Here's how the part is built. I have some questions about the finished solid (model axes, mm). A direction names the side the tool comes from. Coordinates: 2 decimals unless noted, no trailing zeros. Order: outer loops, then holes, each group sorted by start corner. A loop starts at its lowest first (then second) coordinate and runs counter-clockwise, first axis right, second up. Notation, with made-up numbers: (-26.75, 65.5) - (9.25, 65.5) arc R8 ccw to (9.25, 76.5) - close; hole circle Ø11 at (6, -33). An arc over 180 degrees is marked (long way). Answer as CSV lines item,"result". Start each with the question number.
Item 1: Imagine slicing it at D-D on x = -48. List the corners of the cut face in (y, z) for me.
Item 2: Imagine slicing it at C-C on z = -21. List the corners of the cut face in (x, y) for me (3 decimals), and give its area (3 significant figures).
Item 3: I need wall thicknesses on line 1 (X direction, y = -0.4, z = 0); line 2 (X direction, y = -0.65, z = -41); line 3 (Y direction, x = 40, z = -75.5). Which ranges of each line are inside material? Lowest first, please.
Item 4: On a 3-axis mill with a long thin cutter (end or side, diameter ignored), from which of +Z, -Z, +X, -X, +Y, -Y can I reach the whole of each face in a straight line? I mean faces 4 (the face through (83.647, -0.986, 7.831)), 5 (the face through (28.5, -1.49, -29.57)). Say none if no direction works.
Item 5: I'm going to push flat-ended pins straight in: pin 1 (0.8 mm diameter, centred on x = 22, z = -25, fed in from -Y) (3 decimals); pin 2 (12 mm diameter, centred on x = 11, z = -55.5, fed in from +Y); pin 3 (19 mm diameter, centred on x = -15.5, z = 22, fed in from -Y); pin 4 (0.5 mm diameter, centred on y = -1.5, z = 23, fed in from +X). Where does each tip first touch, or does it pass through?
Item 6: We'd pull the mould along Z, two halves only. Please class faces 1 (the face through (3.167, -0.986, -89.444)), 2 (the face through (7.509, -0.493, 23.846)), 3 (the face through (-28.57, -1.49, -29.5)): pulls with the +Z half, pulls with the -Z half, needs draft (parallel to the pull), parting line crosses it, or undercut.
Item 7: Imagine slicing it at A-A on x = 0. List the corners of the cut face in (y, z) for me.
Item 8: Imagine slicing it at B-B on z = -47.5. List the corners of the cut face in (x, y) for me.
from build123d import *

# Parameters (mm, degrees)
BOSS_EXTRUDE1_DEPTH = 2
SKETCH9_R           = 5.15
CUT_EXTRUDE3_DEPTH  = 127.587914115
VISION_PATTERN_R    = 25
VISION_PATTERN_R_2  = 20
CUT_EXTRUDE4_DEPTH  = 127.587914115
FILLET1_R           = 10
BOSS_EXTRUDE4_DEPTH = 50
SKETCH12_W          = 60
SKETCH12_H          = 106
CUT_EXTRUDE5_DEPTH  = 1
SKETCH16_R          = 12.5
CUT_EXTRUDE9_DEPTH  = 20
SKETCH17_R          = 0.75
BOSS_EXTRUDE3_DEPTH = 0.425
CHAMFER1_SIZE       = 1.8
CHAMFER1_SIZE_2     = 3.860112457
CHAMFER2_SIZE       = 0.987120775
CHAMFER2_SIZE_2     = 1
FILLET3_R           = 0.1
FILLET2_R           = 0.4
FILLET4_R           = 5
FILLET5_R           = 2


with BuildPart() as part:
    # Sketch1 → Boss-Extrude1 (new body)
    with BuildSketch(Plane(origin=(0, 0, 0), x_dir=(1, 0, 0), z_dir=(0, 1, 0))):
        with BuildLine():
            Line((-48.839021284, -75), (48.839021284, -75))
            ThreePointArc((48.839021284, -75), (0, 89.5), (-48.839021284, -75))
        make_face()
    extrude(amount=-BOSS_EXTRUDE1_DEPTH)

    # Sketch9 → Cut-Extrude3 (cut, through all)
    with BuildSketch(Plane(origin=(0, 0, 0), x_dir=(1, 0, 0), z_dir=(0, 1, 0))):
        with Locations(Location((78.541209232, -8.501673503, 0), (0, 0, 270))):
            Circle(SKETCH9_R)
        with Locations(Location((-78.541209232, -8.501673503, 0), (0, 0, 270))):
            Circle(SKETCH9_R)
    extrude(amount=-CUT_EXTRUDE3_DEPTH, mode=Mode.SUBTRACT)

    # Vision Pattern → Cut-Extrude4 (cut, through all)
    with BuildSketch(Plane(origin=(0, 0, 0), x_dir=(1, 0, 0), z_dir=(0, 1, 0))):
        with Locations(Location((0, 0, 0), (0, 0, 270))):
            Circle(VISION_PATTERN_R)
        with Locations(Location((54.772255751, -35, 0), (0, 0, 270))):
            Circle(VISION_PATTERN_R_2)
        with Locations(Location((-54.772255751, -35, 0), (0, 0, 270))):
            Circle(VISION_PATTERN_R_2)
        with Locations(Location((35, 54.772255751, 0), (0, 0, 270))):
            Circle(VISION_PATTERN_R_2)
        with Locations(Location((-35, 54.772255751, 0), (0, 0, 270))):
            Circle(VISION_PATTERN_R_2)
    extrude(amount=-CUT_EXTRUDE4_DEPTH, mode=Mode.SUBTRACT)

    # Fillet1
    fillet1_edges = [part.edges().sort_by_distance(p)[0] for p in [
        (48.839021284, -1, 75),
        (-48.839021284, -1, 75),
    ]]
    fillet(fillet1_edges, radius=FILLET1_R)

    # Sketch18 → Boss-Extrude4 (add)
    with BuildSketch(Plane.XY.offset(5)):
        Polygon((62.854667939, -3.6), (67.145332061, -3.6), (66.025, -2), (63.975, -2), align=None)
    boss_extrude4 = extrude(amount=-BOSS_EXTRUDE4_DEPTH)

    # Mirror2: Boss-Extrude4 across plane
    add(boss_extrude4.mirror(Plane(origin=(0, 0, 0), x_dir=(0, 0, 1), z_dir=(1, 0, 0))))

    # Sketch12 → Cut-Extrude5 (cut)
    with BuildSketch(Plane.XZ.offset(2)):
        with Locations((0, 22)):
            Rectangle(SKETCH12_W, SKETCH12_H)
    extrude(amount=-CUT_EXTRUDE5_DEPTH, mode=Mode.SUBTRACT)

    # Sketch16 → Cut-Extrude9 (cut)
    with BuildSketch(Plane(origin=(0, 0, 0), x_dir=(1, 0, 0), z_dir=(0, 1, 0))):
        with Locations((0, -75)):
            Circle(SKETCH16_R)
    extrude(amount=-CUT_EXTRUDE9_DEPTH, mode=Mode.SUBTRACT)

    # Sketch17 → Boss-Extrude3 (add)
    with BuildSketch(Plane.XZ.offset(1)):
        with Locations(Location((-22, -25, 0), (0, 0, 270))):
            Circle(SKETCH17_R)
    boss_extrude3 = extrude(amount=BOSS_EXTRUDE3_DEPTH)

    # Mirror1: Boss-Extrude3 across plane
    add(boss_extrude3.mirror(Plane(origin=(0, 0, 0), x_dir=(0, 0, 1), z_dir=(1, 0, 0))))

    # Chamfer1
    # the kernel refuses this chamfer: 3.860112457, 1.8 mm, written as the material it takes off along each edge
    with BuildSketch(Plane(origin=(52.853211246, -3.6, -45), x_dir=(0, 0.9971975577536774, -0.07481330637060049), z_dir=(1, 0, 0))) as chamfer1_piece_1_section:
        Polygon((CHAMFER1_SIZE * 0.997197557754, CHAMFER1_SIZE * 0.0748133063706), (-CHAMFER1_SIZE_2 * 0.074813306369, CHAMFER1_SIZE_2 * 0.997197557732), (0, 0), align=None)
    chamfer1_piece_1 = extrude(amount=24.293577508, mode=Mode.PRIVATE)
    chamfer1_piece_1 = split(chamfer1_piece_1, bisect_by=Plane(origin=(65, -2, -43.665311996), z_dir=(0, -1, 0)), keep=Keep.TOP, mode=Mode.PRIVATE)
    add(chamfer1_piece_1, mode=Mode.SUBTRACT)
    with BuildSketch(Plane(origin=(52.853211246, -3.6, 5), x_dir=(0, 0.9971975577536774, 0.07481330637060049), z_dir=(1, 0, 0))) as chamfer1_piece_2_section:
        Polygon((CHAMFER1_SIZE * 0.997197557754, -CHAMFER1_SIZE * 0.0748133063706), (-CHAMFER1_SIZE_2 * 0.074813306369, -CHAMFER1_SIZE_2 * 0.997197557732), (0, 0), align=None)
    chamfer1_piece_2 = extrude(amount=24.293577508, mode=Mode.PRIVATE)
    chamfer1_piece_2 = split(chamfer1_piece_2, bisect_by=Plane(origin=(65, -2, 3.665311996), z_dir=(0, -1, 0)), keep=Keep.TOP, mode=Mode.PRIVATE)
    add(chamfer1_piece_2, mode=Mode.SUBTRACT)
    with BuildSketch(Plane(origin=(-52.853211246, -3.6, 5), x_dir=(0, 0.9971975577536774, 0.07481330637060049), z_dir=(-1, 0, 0))) as chamfer1_piece_3_section:
        Polygon((CHAMFER1_SIZE * 0.997197557754, CHAMFER1_SIZE * 0.0748133063706), (-CHAMFER1_SIZE_2 * 0.074813306369, CHAMFER1_SIZE_2 * 0.997197557732), (0, 0), align=None)
    chamfer1_piece_3 = extrude(amount=24.293577508, mode=Mode.PRIVATE)
    chamfer1_piece_3 = split(chamfer1_piece_3, bisect_by=Plane(origin=(-65, -2, 3.665311996), z_dir=(0, -1, 0)), keep=Keep.TOP, mode=Mode.PRIVATE)
    add(chamfer1_piece_3, mode=Mode.SUBTRACT)
    with BuildSketch(Plane(origin=(-52.853211246, -3.6, -45), x_dir=(0, 0.9971975577536774, -0.07481330637060049), z_dir=(-1, 0, 0))) as chamfer1_piece_4_section:
        Polygon((CHAMFER1_SIZE * 0.997197557754, -CHAMFER1_SIZE * 0.0748133063706), (-CHAMFER1_SIZE_2 * 0.074813306369, -CHAMFER1_SIZE_2 * 0.997197557732), (0, 0), align=None)
    chamfer1_piece_4 = extrude(amount=24.293577508, mode=Mode.PRIVATE)
    chamfer1_piece_4 = split(chamfer1_piece_4, bisect_by=Plane(origin=(-65, -2, -43.665311996), z_dir=(0, -1, 0)), keep=Keep.TOP, mode=Mode.PRIVATE)
    add(chamfer1_piece_4, mode=Mode.SUBTRACT)

    # Chamfer2
    # the kernel refuses this chamfer: 1, 0.987120775 mm, written as the material it takes off along each edge
    with BuildSketch(Plane(origin=(-65.301002381, -0.966024243, 6.788466782), x_dir=(0.4696180134880429, 0.7314458045546072, -0.49441476151810837), z_dir=(-0.2837570390591316, -0.4052470497313357, -0.8690551026652124))) as chamfer2_piece_1_section:
        Polygon((CHAMFER2_SIZE * 0.999392501434, CHAMFER2_SIZE * 0.0348515221858), (CHAMFER2_SIZE_2 * 0.489748534071, CHAMFER2_SIZE_2 * 0.871863735555), (0, 0), align=None)
    chamfer2_piece_1 = extrude(amount=9.051149208, mode=Mode.PRIVATE)
    chamfer2_piece_1 = split(chamfer2_piece_1, bisect_by=Plane(origin=(-66.526786639, -2, 1.318548556), z_dir=(0, -1, 0)), keep=Keep.TOP, mode=Mode.PRIVATE)
    add(chamfer2_piece_1, mode=Mode.SUBTRACT)
    with BuildSketch(Plane(origin=(-62.13067032, -4.633975757, -1.077480623), x_dir=(-0.46961801348803994, 0.73144580455461, -0.49441476151810687), z_dir=(-0.28375703905912847, 0.40524704973133613, 0.8690551026652132))) as chamfer2_piece_2_section:
        Polygon((CHAMFER2_SIZE * 0.999392501434, CHAMFER2_SIZE * 0.0348515221858), (CHAMFER2_SIZE_2 * 0.489748534071, CHAMFER2_SIZE_2 * 0.871863735555), (0, 0), align=None)
    chamfer2_piece_2 = extrude(amount=9.051149208, mode=Mode.PRIVATE)
    chamfer2_piece_2 = split(chamfer2_piece_2, bisect_by=Plane(origin=(-63.473213361, -2, 1.318548556), z_dir=(0, -1, 0)), keep=Keep.TOP, mode=Mode.PRIVATE)
    add(chamfer2_piece_2, mode=Mode.SUBTRACT)
    with BuildSketch(Plane(origin=(64.698997619, -0.966024243, 6.788466782), x_dir=(0.9583436918926346, -0.15061389857445218, -0.24267843284024973), z_dir=(-0.28375703905912847, -0.40524704973133613, -0.8690551026652132))) as chamfer2_piece_3_section:
        Polygon((CHAMFER2_SIZE_2 * 0.999423797129, -CHAMFER2_SIZE_2 * 0.0339422116651), (CHAMFER2_SIZE * 0.490541595675, -CHAMFER2_SIZE * 0.871417777782), (0, 0), align=None)
    chamfer2_piece_3 = extrude(amount=9.051149208, mode=Mode.PRIVATE)
    chamfer2_piece_3 = split(chamfer2_piece_3, bisect_by=Plane(origin=(63.473213361, -2, 1.318548556), z_dir=(0, -1, 0)), keep=Keep.TOP, mode=Mode.PRIVATE)
    add(chamfer2_piece_3, mode=Mode.SUBTRACT)
    with BuildSketch(Plane(origin=(67.86932968, -4.633975757, -1.077480623), x_dir=(-0.46961801348803955, 0.7314458045546093, -0.4944147615181082), z_dir=(-0.2837570390591316, 0.4052470497313357, 0.8690551026652124))) as chamfer2_piece_4_section:
        Polygon((CHAMFER2_SIZE * 0.999392501434, CHAMFER2_SIZE * 0.0348515221858), (CHAMFER2_SIZE_2 * 0.489748534071, CHAMFER2_SIZE_2 * 0.871863735555), (0, 0), align=None)
    chamfer2_piece_4 = extrude(amount=9.051149208, mode=Mode.PRIVATE)
    chamfer2_piece_4 = split(chamfer2_piece_4, bisect_by=Plane(origin=(66.526786639, -2, 1.318548556), z_dir=(0, -1, 0)), keep=Keep.TOP, mode=Mode.PRIVATE)
    add(chamfer2_piece_4, mode=Mode.SUBTRACT)
    with BuildSketch(Plane(origin=(-65.301002381, -0.966024243, -46.788466782), x_dir=(0.46961801348803894, 0.7314458045546097, 0.49441476151810826), z_dir=(-0.2837570390591316, -0.4052470497313357, 0.8690551026652124))) as chamfer2_piece_5_section:
        Polygon((CHAMFER2_SIZE * 0.999392501434, -CHAMFER2_SIZE * 0.0348515221858), (CHAMFER2_SIZE_2 * 0.489748534071, -CHAMFER2_SIZE_2 * 0.871863735555), (0, 0), align=None)
    chamfer2_piece_5 = extrude(amount=9.051149208, mode=Mode.PRIVATE)
    chamfer2_piece_5 = split(chamfer2_piece_5, bisect_by=Plane(origin=(-66.526786639, -2, -41.318548556), z_dir=(0, -1, 0)), keep=Keep.TOP, mode=Mode.PRIVATE)
    add(chamfer2_piece_5, mode=Mode.SUBTRACT)
    with BuildSketch(Plane(origin=(-62.13067032, -4.633975757, -38.922519377), x_dir=(-0.46961801348803905, 0.7314458045546104, 0.49441476151810687), z_dir=(-0.28375703905912847, 0.40524704973133613, -0.8690551026652132))) as chamfer2_piece_6_section:
        Polygon((CHAMFER2_SIZE * 0.999392501434, -CHAMFER2_SIZE * 0.0348515221858), (CHAMFER2_SIZE_2 * 0.489748534071, -CHAMFER2_SIZE_2 * 0.871863735555), (0, 0), align=None)
    chamfer2_piece_6 = extrude(amount=9.051149208, mode=Mode.PRIVATE)
    chamfer2_piece_6 = split(chamfer2_piece_6, bisect_by=Plane(origin=(-63.473213361, -2, -41.318548556), z_dir=(0, -1, 0)), keep=Keep.TOP, mode=Mode.PRIVATE)
    add(chamfer2_piece_6, mode=Mode.SUBTRACT)
    with BuildSketch(Plane(origin=(64.698997619, -0.966024243, -46.788466782), x_dir=(0.9583436918926347, -0.150613898574452, 0.24267843284024984), z_dir=(-0.28375703905912847, -0.40524704973133613, 0.8690551026652132))) as chamfer2_piece_7_section:
        Polygon((CHAMFER2_SIZE_2 * 0.999423797129, CHAMFER2_SIZE_2 * 0.0339422116651), (CHAMFER2_SIZE * 0.490541595675, CHAMFER2_SIZE * 0.871417777782), (0, 0), align=None)
    chamfer2_piece_7 = extrude(amount=9.051149208, mode=Mode.PRIVATE)
    chamfer2_piece_7 = split(chamfer2_piece_7, bisect_by=Plane(origin=(63.473213361, -2, -41.318548556), z_dir=(0, -1, 0)), keep=Keep.TOP, mode=Mode.PRIVATE)
    add(chamfer2_piece_7, mode=Mode.SUBTRACT)
    with BuildSketch(Plane(origin=(67.86932968, -4.633975757, -38.922519377), x_dir=(-0.46961801348803994, 0.731445804554609, 0.49441476151810815), z_dir=(-0.2837570390591316, 0.4052470497313357, -0.8690551026652124))) as chamfer2_piece_8_section:
        Polygon((CHAMFER2_SIZE * 0.999392501434, -CHAMFER2_SIZE * 0.0348515221858), (CHAMFER2_SIZE_2 * 0.489748534071, -CHAMFER2_SIZE_2 * 0.871863735555), (0, 0), align=None)
    chamfer2_piece_8 = extrude(amount=9.051149208, mode=Mode.PRIVATE)
    chamfer2_piece_8 = split(chamfer2_piece_8, bisect_by=Plane(origin=(66.526786639, -2, -41.318548556), z_dir=(0, -1, 0)), keep=Keep.TOP, mode=Mode.PRIVATE)
    add(chamfer2_piece_8, mode=Mode.SUBTRACT)

    # Fillet3
    fillet3_edges = [part.edges().sort_by_distance(p)[0] for p in [
        (-67.145332061, -3.6, -20),
        (-65, -3.6, -41.139887543),
        (-62.854667939, -3.6, -20),
        (-65, -3.6, 1.139887543),
        (-63.376100806, -3.6, 0.142222043),
        (-66.623899194, -3.6, 0.142222043),
        (-63.376100806, -3.6, -40.142222043),
        (-66.623899194, -3.6, -40.142222043),
        (62.854667939, -3.6, -20),
        (65, -3.6, -41.139887543),
        (67.145332061, -3.6, -20),
        (65, -3.6, 1.139887543),
        (66.623899194, -3.6, 0.142222043),
        (63.376100806, -3.6, 0.142222043),
        (66.623899194, -3.6, -40.142222043),
        (63.376100806, -3.6, -40.142222043),
    ]]
    fillet(fillet3_edges, radius=FILLET3_R)

    # Fillet2
    fillet2_edges = [part.edges().sort_by_distance(p)[0] for p in [
        (-22, -1.425, -24.25),
        (22, -1.425, -24.25),
    ]]
    fillet(fillet2_edges, radius=FILLET2_R)

    # Fillet4
    fillet4_edges = [part.edges().sort_by_distance(p)[0] for p in [
        (-30, -1.5, -31),
        (30, -1.5, -31),
    ]]
    fillet(fillet4_edges, radius=FILLET4_R)

    # Fillet5
    fillet5_edges = [part.edges().sort_by_distance(p)[0] for p in [
        (-12.5, -0.5, 75),
        (-30, -1.5, 75),
        (30, -1.5, 75),
        (12.5, -0.5, 75),
    ]]
    fillet(fillet5_edges, radius=FILLET5_R)


solid = part.part
Responses:
1,outline,"(-2, -75.54) - (0, -75.54) - (0, -69.97) - (-2, -69.97) - close; (-2, -39.57) - (0, -39.57) - (0, 16.18) - (-2, 16.18) - close; (-2, 53.82) - (0, 53.82) - (0, 74.75) - (-2, 74.75) - close"
2,outline,"(-87.001, -2) - (-66.025, -2) - (-67.035, -3.443) arc R0.1 ccw to (-66.953, -3.6) - (-63.047, -3.6) arc R0.1 ccw to (-62.965, -3.443) - (-63.975, -2) - (-30, -2) - (-30, -1) - (-13.565, -1) - (-13.565, 0) - (-87.001, 0) - close; (13.565, -1) - (30, -1) - (30, -2) - (63.975, -2) - (62.965, -3.443) arc R0.1 ccw to (63.047, -3.6) - (66.953, -3.6) arc R0.1 ccw to (67.035, -3.443) - (66.025, -2) - (87.001, -2) - (87.001, 0) - (13.565, 0) - close"
2,area,"271 mm^2"
3,line 1,"x = -89.5 to -25, 25 to 89.5"
3,line 2,"x = -79.56 to -49.5, -20.5 to 20.5, 49.5 to 79.56"
3,line 3,"y = -2 to 0"
4,face 4,"+Y, -Y"
4,face 5,"+Z, -Y"
5,pin 1,"stops at y = -1.425"
5,pin 2,"stops at y = 0"
5,pin 3,"stops at y = -1"
5,pin 4,"stops at x = 86.56"
6,face 1,"parting line crosses it"
6,face 2,"undercut"
6,face 3,"pulls with the +Z half"
7,outline,"(-2, -89.5) - (0, -89.5) - (0, -25) - (-1, -25) - (-1, -31) - (-2, -31) - close; (-1, 25) - (0, 25) - (0, 62.5) - (-1, 62.5) - close"
8,outline,"(-75.86, -2) - (-53.63, -2) - (-53.63, 0) - (-75.86, 0) - close; (-16.37, -2) - (16.37, -2) - (16.37, 0) - (-16.37, 0) - close; (53.63, -2) - (75.86, -2) - (75.86, 0) - (53.63, 0) - close"
